Autodesk Inventor part; units mm, degrees
ref_plane "YZ Plane" through (0, 0, 0) normal (1, 0, 0) x (0, 1, 0)
ref_plane "XZ Plane" through (0, 0, 0) normal (0, 1, 0) x (-1, 0, 0)
ref_plane "XY Plane" through (0, 0, 0) normal (0, 0, 1) x (1, 0, 0)
sketch "Esboço1" plane through (0, 0, 0) normal (0, 1, 0) x (-1, 0, 0)
  circle A0 centre (0, 0) radius 4
  dimension "d0" = 8
extrude "Extrusão1" add sketch "Esboço1" along normal blind 21
fillet "Arredondamento1" radius 4 1 edges at (4, 0, 0)
sketch "Esboço2" plane through (0, 21, 0) normal (0, 1, 0) x (1, 0, 0)
  point P0 (0, 0)
  point P1 (0, 0)
hole "Furo1" at (0, 21, 0) direction (0, -1, 0) diameter 3.242 depth 10
properties part number "Dedo-02"
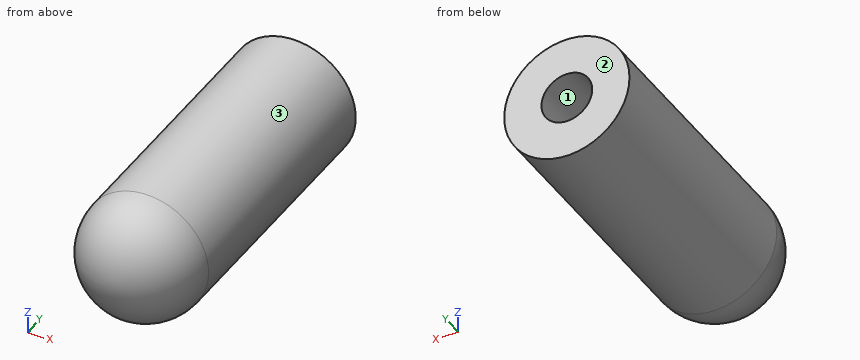
Design review of the part built by this model. Coordinates are the model's own, in mm. Face numbers are marked on the shaded views. Give positions to 0.01 mm unless a question says otherwise; leave off trailing zeros. Order: outer loops, then holes, each group sorted by start corner. A loop starts at its lowest first (then second) coordinate and runs counter-clockwise, first axis right, second up. Notation, with made-up numbers: (72.25, -1) - (94.25, -1) arc R17 cw to (94.25, 9) - close; hole circle Ø3 at (5, 42.25). An arc over 180 degrees is marked (long way). Use a Markdown table: item, result. Add a question column.
(1) Clearance check with flat-ended pins moving along their axes: P1, Ø1.5, axis at x = 1, y = 4.5, coming from the -Z side; P2, Ø1.5, axis at y = 11, z = -1.5, coming from the -X side; P3, Ø1.5, axis at x = -0.5, z = 0.5, coming from the +Y side. State where each tip first meets the part, or that it passes through.
(2) Add section A-A on z = 0. Give the boundary of the cut face in (x, y), then the cut area to 3 significant figures.
(3) Add section D-D on y = 10. Give the boundary of the cut face in (x, z).
(4) Add section C-C on y = 14.5. Give the boundary of the cut face in (x, z).
(5) Mouldability with a two-part tool opening along Z and no side actions: class the marked faces 1, 2 and 3 as +Z half, -Z half, draft (parallel to the pull), parting line (faces both ways), or undercut.
(6) Wall thickness on probe 1 along Z at (x, y) = (0, 16); probe 2 along X at (y, z) = (15, 0.25); probe 3 along Z at (x, y) = (1.75, 3.25): over which ranges is each line inside the solid? List them lowest first. Write a range as [from, to].
(7) Add section B-B on x = 0. Give the boundary of the cut face in (y, z), then the cut area to 3 significant figures.
Report:
| question | item | result |
|---|---|---|
| 1 | P1 | stops at z = -3.99 |
| 1 | P2 | stops at x = -3.93 |
| 1 | P3 | stops at y = 11 |
| 2 | outline | (-4, 4) arc R4 ccw to (4, 4) - (4, 21) - (1.62, 21) - (1.62, 11) - (-1.62, 11) - (-1.62, 21) - (-4, 21) - close |
| 2 | area | 129 mm² |
| 3 | outline | circle Ø8 at (0, 0) |
| 4 | outline | circle Ø8 at (0, 0); hole circle Ø3.24 at (0, 0) |
| 5 | face 1 | undercut |
| 5 | face 2 | draft |
| 5 | face 3 | parting line |
| 6 | probe 1 | z = [-4, -1.62], [1.62, 4] |
| 6 | probe 2 | x = [-3.99, -1.6], [1.6, 3.99] |
| 6 | probe 3 | z = [-3.52, 3.52] |
| 7 | outline | (4, -4) - (21, -4) - (21, -1.62) - (11, -1.62) - (11, 1.62) - (21, 1.62) - (21, 4) - (4, 4) arc R4 ccw to start |
| 7 | area | 129 mm² |
